from build123d import *

# Parameters (mm, degrees)
F0_W           = 10
F0_H           = 14
F1_DEPTH       = 5.5
F4_D           = 2.83
F4_CBORE_D     = 5.9
F4_CBORE_DEPTH = 2.2
F2_W           = 8
F2_H           = 1.5
F5_DEPTH       = 11
F6_SIZE        = 1
F7_R           = 1
F8_T4_DEPTH    = 1.5
F9_SIZE        = 0.49999
F10_R          = 0.5


# Not quite as in the source:
# - a fillet or chamfer that OpenCascade refuses, or shapes differently, is made with other operations: its cross-section is extruded or revolved along the edge and cut away or added
# - a fillet or chamfer is up to 0.001 mm smaller than in the source, because OpenCascade refuses the exact size


with BuildPart() as f1:
    # F0 (on Top) → F1 (new body)
    with BuildSketch(Plane.XY):
        with Locations((5, 7)):
            Rectangle(F0_W, F0_H)
    extrude(amount=F1_DEPTH)

    # F4 (through all)
    with Locations(Plane.XY.offset(5.5)):
        with Locations((5, 9)):
            CounterBoreHole(F4_D / 2, F4_CBORE_D / 2, F4_CBORE_DEPTH)

    # F2 (on Top) → F5 (join)
    with BuildSketch(Plane.XY):
        with Locations((3, 3.25)):
            Rectangle(F2_W, F2_H)
    extrude(amount=F5_DEPTH)

    # F6
    f6_edges = [f1.edges().sort_by_distance(p)[0] for p in [
        (-1, 3.25, 0),
    ]]
    chamfer(f6_edges, length=F6_SIZE)

    # F7
    f7_edges = [f1.edges().sort_by_distance(p)[0] for p in [
        (0, 14, 2.75),
        (10, 14, 2.75),
        (10, 0, 2.75),
        (0, 0, 2.75),
    ]]
    fillet(f7_edges, radius=F7_R)

    # F8: chamfer of 5 on 1 edges, made by hand


with BuildPart() as f8_tool2:
    # F8_s3 → F8_t4 (new body)
    with BuildSketch(Plane.XZ.offset(-4)):
        Polygon((12, 5.5), (7, 10.5), (7, 5.5), align=None)
    extrude(amount=F8_T4_DEPTH)

    split(bisect_by=Plane.YZ.offset(10), keep=Keep.BOTTOM)


with BuildPart() as f1_1:
    add(f1.part)

    # F8_t1: union F8_tool2
    add(f8_tool2.part)

    # F9 (size 0.5 in the source; OpenCascade refuses exactly that, so slightly less here)
    f9_edges = [f1_1.edges().sort_by_distance(p)[0] for p in [
        (7, 3.25, 11),
    ]]
    chamfer(f9_edges, length=F9_SIZE)

    # F10
    f10_edges = [f1_1.edges().sort_by_distance(p)[0] for p in [
        (5, 4, 5.5),
        (5, 2.5, 5.5),
    ]]
    fillet(f10_edges, radius=F10_R)


solid = f1_1.part
Part model, mm, in its own coordinate system. A direction names the side the tool comes from. Coordinates: 2 decimals unless noted, no trailing zeros. Write each loop counter-clockwise with the first axis right and the second up, starting at its lowest first coordinate (ties: lowest second). Pieces come first, ordered by that corner, then holes. Notation, with made-up numbers: (-17, 60.25) - (-2, 60.25) arc R27 ccw to (-2, 96.25) - close; hole circle Ø8 at (21.25, -37). An arc over 180 degrees is marked (long way). Put each result on its own line as item: value.
1. Band-saw the part on C-C (z = 2.25). Write the cut outline in (x, y) (3 decimals).
Final values:
outline: (-1, 2.5) - (0, 2.5) - (0, 1) arc R1 ccw to (1, 0) - (9, 0) arc R1 ccw to (10, 1) - (10, 13) arc R1 ccw to (9, 14) - (1, 14) arc R1 ccw to (0, 13) - (0, 4) - (-1, 4) - close; hole circle Ø2.83 at (5, 9)
2. Probe line 1 along Y through (x, z) = (5, 5); line 2 along Z through (x, y) = (1, 8.5); line 3 along Y through (x, z) = (2.25, 7.75). List the from-to ranges inside material, lowest first. Write a range as [from, to].
Final values:
line 1: y = [0, 6.05], [11.95, 14]
line 2: z = [0, 5.5]
line 3: y = [2.5, 4]
3. Band-saw the part on D-D (x = 8.25). Write the cut outline in (y, z), then the cut area to 3 significant figures.
Final values:
outline: (0, 0) - (14, 0) - (14, 5.5) - (4.5, 5.5) arc R0.5 cw to (4, 6) - (4, 9.25) - (2.5, 9.25) - (2.5, 6) arc R0.5 cw to (2, 5.5) - (0, 5.5) - close
area: 82.7 mm²
4. Band-saw the part on A-A (y = 9). Write the cut outline in (x, z) (3 decimals), then the cut area to 3 significant figures.
Final values:
outline: (0, 0) - (3.585, 0) - (3.585, 3.3) - (2.05, 3.3) - (2.05, 5.5) - (0, 5.5) - close; (6.415, 0) - (10, 0) - (10, 5.5) - (7.95, 5.5) - (7.95, 3.3) - (6.415, 3.3) - close
area: 32.7 mm²
5. Flat gauge pins, fed straight in: pin 1 Ø3.5 at (x, y) = (5, 9) entering from +Z; pin 2 Ø1.5 at (y, z) = (3, 8.5) entering from +X; pin 3 Ø0.5 at (y, z) = (1.5, 2.5) entering from -X. Where does each tip first touch, or does it go through?
Final values:
pin 1: stops at z = 3.3
pin 2: stops at x = 9.75
pin 3: stops at x = 0
6. Band-saw the part on B-B (x = 5). Write the cut outline in (y, z) (3 decimals), then the cut area to 3 significant figures.
Final values:
outline: (0, 0) - (7.585, 0) - (7.585, 3.3) - (6.05, 3.3) - (6.05, 5.5) - (4.5, 5.5) arc R0.5 cw to (4, 6) - (4, 11) - (2.5, 11) - (2.5, 6) arc R0.5 cw to (2, 5.5) - (0, 5.5) - close; (10.415, 0) - (14, 0) - (14, 5.5) - (11.95, 5.5) - (11.95, 3.3) - (10.415, 3.3) - close
area: 63.0 mm²
7. Two-plate mould, pull along Y, no slides. Class faces 1 (the flat face through (5, 0, 3)), 2 (the flat face through (5, 1, 5.5)), 3 (the cylindrical face through (5.2, 10.4, 1.6)), 4 (the cylindrical face through (6.586, 11.487, 4.415)): +Y half, -Y half, draft (parallel to the pull), parting line (faces both ways), or undercut.
Final values:
face 1: -Y half
face 2: draft
face 3: undercut
face 4: undercut
8. 3-axis set-ups, long thin cutter, end or side, ignore diameter. For faces 5 (the flat face through (4.3, 10.4, 3.3)), 6 (the flat face through (0, 8, 2)), 7 (the flat face through (2.7, 11.4, 5.5)): which of +Z, -Z, +X, -X, +Y, -Y reach the whole face in a straight line?
Final values:
face 5: +Z
face 6: +Z, -Z, -X, +Y
face 7: +Z, +X, -X, +Y
